from build123d import *

# Parameters (mm, degrees)
BOSS_EXTRUDE1_DEPTH = 80.5


with BuildPart() as part:
    # Sketch1 → Boss-Extrude1 (new body)
    with BuildSketch(Plane.XY):
        with BuildLine():
            Line((-22.496419286, 29.27), (-22.496419286, 10))
            ThreePointArc((-22.496419286, 10), (-19.567487097, 2.928932188), (-12.496419286, 0))
            Line((-12.496419286, 0), (36.648732275, 0))
            ThreePointArc((36.648732275, 0), (43.719800087, 2.928932188), (46.648732275, 10))
            Line((46.648732275, 10), (46.648732275, 29.27))
            Line((46.648732275, 29.27), (38.088732275, 29.27))
            Line((38.088732275, 29.27), (38.088732275, 17.58))
            Line((38.088732275, 17.58), (35.026959912, 14.518227637))
            Line((35.026959912, 14.518227637), (29.456959912, 14.518227637))
            ThreePointArc((29.456959912, 14.518227637), (12.076156495, 3.858910448), (-5.304646923, 14.518227637))
            Line((-5.304646923, 14.518227637), (-10.874646923, 14.518227637))
            Line((-10.874646923, 14.518227637), (-13.936419286, 17.58))
            Line((-13.936419286, 17.58), (-13.936419286, 29.27))
            Line((-13.936419286, 29.27), (-22.496419286, 29.27))
        make_face()
    extrude(amount=BOSS_EXTRUDE1_DEPTH)


solid = part.part
Work out the finished part from the listing and answer in its coordinate system (mm). A direction names the side the tool comes from. Coordinates: 2 decimals unless noted, no trailing zeros. Loops run counter-clockwise (first coordinate to the right, second up) from the corner with the lowest first, then second, coordinate; pieces in that order, holes last. Notation, with made-up numbers: M 62,77 L 80,77 A27 cw 80,99 Z; hole C 22.25,64.25 d4. An arc over 180 degrees is marked long. Answer in a Markdown table with one row per item. Add a question column.
1. Find section B-B, the plane z = 47. Write down the section's boundary in (x, y).
2. Flat-ended cylindrical pins translate along their axes: P1, Ø2, axis at x = 38, z = 36.5, coming from the -Y side; P2, Ø6, axis at x = 33, z = 29, coming from the +Y side; P3, Ø4, axis at x = 16.5, z = 40.5, coming from the +Y side. Find the tip coordinate at first contact, or state that the pin passes through.
3. Consider L1, parallel to X at y = 23.25, z = 65.5; L2, parallel to X at y = 12.75, z = 52.5; L3, parallel to Y at x = 12, z = 67.5. Determine where each line is inside the solid, lowest interval first.
4. The mould has two halves that part along X. Classify faces 1 (the flat face through (-12.384, 16.028, 39.686)), 2 (the flat face through (12, 2, 0)), 3 (the flat face through (36.58, 16.07, 39.69)), 4 (the cylindrical face through (-19.645, 3.007, 39.686)): pulls with the +X half, pulls with the -X half, needs draft (parallel to the pull), parting line crosses it, or undercut.
5. Find section C-C, the plane y = 12.75. Write down the section's boundary in (x, z), then the cut area to 3 significant figures.
6. A tool of negligible diameter and unlimited length cuts with its end or side. For faces 5 (the flat face through (-8, 14.518, 40)), 6 (the flat face through (46.649, 20, 40)), from which of +Z, -Z, +X, -X, +Y, -Y can it reach the whole face along a straight path? Write none if from no direction.
7. Find section A-A, the plane y = 20. Write down the section's boundary in (x, z), then the cut area to 3 significant figures.
8. Find section D-D, the plane x = -8. Write down the section's boundary in (y, z).
Reported:
| question | item | result |
|---|---|---|
| 1 | outline | M -22.5,10 A10 ccw -12.5,0 L 36.65,0 A10 ccw 46.65,10 L 46.65,29.27 L 38.09,29.27 L 38.09,17.58 L 35.03,14.52 L 29.46,14.52 A19.5 cw -5.3,14.52 L -10.87,14.52 L -13.94,17.58 L -13.94,29.27 L -22.5,29.27 Z |
| 2 | P1 | stops at y = 0.01 |
| 2 | P2 | stops at y = 15.49 |
| 2 | P3 | stops at y = 4.95 |
| 3 | L1 | x = -22.5 to -13.94, 38.09 to 46.65 |
| 3 | L2 | x = -22.5 to -4.29, 28.44 to 46.65 |
| 3 | L3 | y = 0 to 3.86 |
| 4 | face 1 | undercut |
| 4 | face 2 | needs draft |
| 4 | face 3 | undercut |
| 4 | face 4 | pulls with the -X half |
| 5 | outline | M -22.5,0 L -4.29,0 L -4.29,80.5 L -22.5,80.5 Z; M 28.44,0 L 46.65,0 L 46.65,80.5 L 28.44,80.5 Z |
| 5 | area | 2,930 mm^2 |
| 6 | face 5 | +Z, -Z, +Y |
| 6 | face 6 | +Z, -Z, +X, +Y, -Y |
| 7 | outline | M -22.5,0 L -13.94,0 L -13.94,80.5 L -22.5,80.5 Z; M 38.09,0 L 46.65,0 L 46.65,80.5 L 38.09,80.5 Z |
| 7 | area | 1,380 mm^2 |
| 8 | outline | M 0,0 L 14.52,0 L 14.52,80.5 L 0,80.5 Z |
